from build123d import *
from OCP.BRepFilletAPI import BRepFilletAPI_MakeFillet

# Parameters (mm, degrees)
BOSS_EXTRUDE1_DEPTH = 5
BOSS_EXTRUDE2_DEPTH = 6.75
CHAMFER1_SIZE       = 3
CUT_EXTRUDE1_DEPTH  = 51.906134019
FILLET1_R1          = 1
FILLET1_R2          = 4
FILLET2_R           = 4
FILLET3_R           = 2
SKETCH5_R           = 1.25
CUT_EXTRUDE2_DEPTH  = 51.906134019
SKETCH6_R           = 1.25
CUT_EXTRUDE3_DEPTH  = 29.824774908
FILLET4_R           = 2
SKETCH7_R           = 3.5
CUT_EXTRUDE4_DEPTH  = 29.824774908
CHAMFER2_SIZE       = 0.5


with BuildPart() as part:
    # Sketch1 → Boss-Extrude1 (new, symmetric)
    with BuildSketch(Plane.XY):
        Polygon((-15, 33.787773645), (11.504683177, 39.681261814), (11.070572477, 41.63358041), (6.189775987, 40.548303662), (6.298303662, 40.060224013), (5.810224013, 39.951696338), (5.701696338, 40.439775987), (-11.855909094, 36.53572857), (-11.747381419, 36.047648921), (-12.235461068, 35.939121246), (-12.343988743, 36.427200895), (-17, 35.391906601), (-17, 20.3), (-16.5, 20.3), (-16.5, 19.8), (-17, 19.8), (-17, 17.5), (-15, 17.5), align=None)
    extrude(amount=BOSS_EXTRUDE1_DEPTH, both=True)

    # Sketch3 → Boss-Extrude2 (add, symmetric)
    with BuildSketch(Plane.XY):
        Polygon((-6.541001904, 35.668686722), (-6.975112604, 37.621005318), (-11.855909094, 36.53572857), (-11.747381419, 36.047648921), (-12.235461068, 35.939121246), (-12.343988743, 36.427200895), (-17, 35.391906601), (-17, 20.3), (-16.5, 20.3), (-16.5, 19.8), (-17, 19.8), (-17, 17.5), (-15, 17.5), (-15, 33.787773645), align=None)
    extrude(amount=BOSS_EXTRUDE2_DEPTH, both=True)

    # Chamfer1
    # the kernel refuses this chamfer: 3 mm, written as the material it takes off along each edge
    with BuildSketch(Plane(origin=(-4.866409254, 28.137569941, -6.75), x_dir=(0.0268403556117362, 0.005968127111591266, 0.9996219169112968), z_dir=(-0.21705534964808215, 0.9761592980600804, 0))) as chamfer1_piece_1_section:
        Polygon((CHAMFER1_SIZE * 0.999621916911, -CHAMFER1_SIZE * 0.0274958766106), (-CHAMFER1_SIZE * 0.0274958766106, -CHAMFER1_SIZE * 0.999621916911), (0, 0), align=None)
    chamfer1_piece_1 = extrude(amount=17.430097928, mode=Mode.PRIVATE)
    chamfer1_piece_1 = split(chamfer1_piece_1, bisect_by=Plane(origin=(-7.864790055, 36.398756806, -5), z_dir=(0, 0, -1)), keep=Keep.TOP, mode=Mode.PRIVATE)
    add(chamfer1_piece_1, mode=Mode.SUBTRACT)
    with BuildSketch(Plane(origin=(-4.866409254, 28.137569941, 6.75), x_dir=(-0.9757902287376033, -0.2169732846910676, 0.02749587661058649), z_dir=(-0.21705534964808215, 0.9761592980600804, 0))) as chamfer1_piece_2_section:
        Polygon((CHAMFER1_SIZE * 0.999621916911, -CHAMFER1_SIZE * 0.0274958766106), (-CHAMFER1_SIZE * 0.0274958766106, -CHAMFER1_SIZE * 0.999621916911), (0, 0), align=None)
    chamfer1_piece_2 = extrude(amount=17.430097928, mode=Mode.PRIVATE)
    chamfer1_piece_2 = split(chamfer1_piece_2, bisect_by=Plane(origin=(-7.864790055, 36.398756806, 5), z_dir=(0, 0, 1)), keep=Keep.TOP, mode=Mode.PRIVATE)
    add(chamfer1_piece_2, mode=Mode.SUBTRACT)

    # Sketch4 → Cut-Extrude1 (cut, through all)
    with BuildSketch(Plane.ZY.offset(17)):
        Polygon((-6.75, 30), (-3.75, 27), (-3.75, 17.5), (3.75, 17.5), (3.75, 27), (6.75, 30), (6.75, 0), (-6.75, 0), align=None)
    extrude(amount=-CUT_EXTRUDE1_DEPTH, mode=Mode.SUBTRACT)

    # Fillet1: one fillet with a radius per group of edges: ONE call of the kernel's fillet builder (fillet() takes one radius for all edges)
    fillet1_edges_1 = [part.edges().sort_by_distance(p)[0] for p in [
        (-9.686535148, 35.993679971, -6.75),
        (-9.686535148, 35.993679971, 6.75),
        (-16, 30, 6.75),
        (-16, 30, -6.75),
    ]]
    fillet1_edges_2 = [part.edges().sort_by_distance(p)[0] for p in [
        (-7.978256377, 36.373526833, 5),
        (-7.978256377, 36.373526833, -5),
        (-16, 27, -3.75),
        (-16, 27, 3.75),
    ]]
    fillet1 = BRepFilletAPI_MakeFillet(part.part.solid().wrapped)
    for e in fillet1_edges_1:
        fillet1.Add(FILLET1_R1, e.wrapped)
    for e in fillet1_edges_2:
        fillet1.Add(FILLET1_R2, e.wrapped)
    add(Compound.cast(fillet1.Shape()), mode=Mode.REPLACE)

    # Fillet2
    fillet2_edges = [part.edges().sort_by_distance(p)[0] for p in [
        (-15, 33.787773645, 0),
    ]]
    fillet(fillet2_edges, radius=FILLET2_R)

    # Fillet3
    fillet3_edges = [part.edges().sort_by_distance(p)[0] for p in [
        (-16, 17.5, -3.75),
        (-16, 17.5, 3.75),
    ]]
    fillet(fillet3_edges, radius=FILLET3_R)

    # Sketch5 → Cut-Extrude2 (cut, through all)
    with BuildSketch(Plane.ZY.offset(17)):
        with Locations(Location((0, 22.5, 0), (0, 0, 270))):
            Circle(SKETCH5_R)
    extrude(amount=-CUT_EXTRUDE2_DEPTH, mode=Mode.SUBTRACT)

    # Sketch6 → Cut-Extrude3 (cut, through all)
    with BuildSketch(Plane(origin=(-8.299779748, 37.326456989, 0), x_dir=(0.9761592980600814, 0.21705534964807782, 0), z_dir=(-0.21705534964807782, 0.9761592980600814, 0))):
        with Locations(Location((17.343433612, 0, 0), (0, 0, 180))):
            Circle(SKETCH6_R)
    extrude(amount=-CUT_EXTRUDE3_DEPTH, mode=Mode.SUBTRACT)

    # Fillet4
    fillet4_edges = [part.edges().sort_by_distance(p)[0] for p in [
        (11.287627827, 40.657421112, -5),
        (11.287627827, 40.657421112, 5),
    ]]
    fillet(fillet4_edges, radius=FILLET4_R)

    # Sketch7 → Cut-Extrude4 (cut, through all)
    with BuildSketch(Plane(origin=(-8.299779748, 37.326456989, 0), x_dir=(0.9761592980600813, 0.21705534964807838, 0), z_dir=(-0.21705534964807838, 0.9761592980600813, 0))):
        with Locations(Location((8.502484958, 0, 0), (0, 0, 180))):
            Circle(SKETCH7_R)
    extrude(amount=-CUT_EXTRUDE4_DEPTH, mode=Mode.SUBTRACT)

    # Chamfer2
    chamfer2_edges = [part.edges().sort_by_distance(p)[0] for p in [
        (3.850668243, 37.979341962, 0),
        (3.416557543, 39.931660559, 0),
    ]]
    chamfer(chamfer2_edges, length=CHAMFER2_SIZE)


solid = part.part
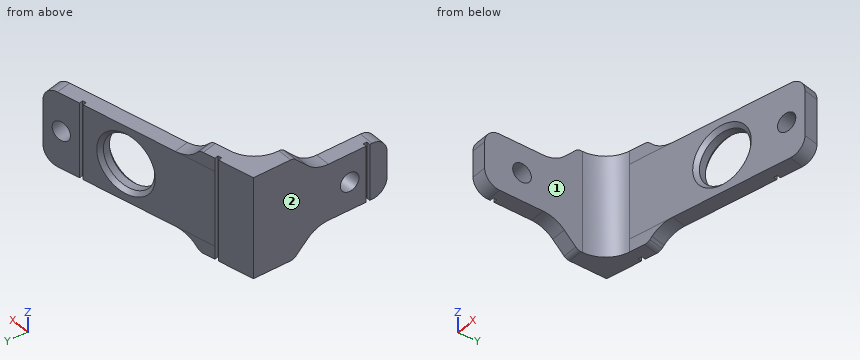
Source: CAD feature listing. Evaluate the final solid. Frame: model axes, mm. Face numbers are marked on the shaded views. A direction names the side the tool comes from. Round coordinates to 2 decimals unless told otherwise and drop trailing zeros. Loops run counter-clockwise (first coordinate to the right, second up) from the corner with the lowest first, then second, coordinate; pieces in that order, holes last. Notation, with made-up numbers: M 80.5,-19.75 L 100.5,-19.75 A15 cw 100.5,-11.75 Z; hole C 22,-13 d7. An arc over 180 degrees is marked long. Return JSON: item names as keys, results as strings. Group by question number.
1. Section query C-C on y = 29.25. Output: boundary loops of the cut face in (x, z).
2. Section query A-A on y = 22.5. Output: boundary loops of the cut face in (x, z), and give its area (3 significant figures).
3. Material intervals for line 1 along Z through (x, y) = (-16.2, 22.5); line 2 along X through (y, z) = (18.75, 2.25); line 3 along Y through (x, z) = (9.25, -2.25), sorted ascending. Write a range as from..to.
4. Pin query (flat end, axial travel): pin 1 (2 mm diameter, centred on x = -5, z = -1.5, fed in from +Y); pin 2 (1.6 mm diameter, centred on x = 4, y = 37.5, fed in from +Z); pin 3 (8 mm diameter, centred on x = -9, z = 5, fed in from +Y). Return the tip coordinate at first contact, or that it passes through.
5. Section query B-B on x = -10.75. Output: boundary loops of the cut face in (y, z), and give its area (3 significant figures).
6. Reachability of the marked faces 1 and 2 from +Z, -Z, +X, -X, +Y, -Y: full face, straight path, thin tool, end or side. Return the list, or none.
7. Section query D-D on z = 0. State how many separate pieces and enclosed holes the cut face has, and give its area (3 significant figures).
Checks:
{
 "1": {"outline": "M -17,-6 L -15,-6 L -15,6 L -17,6 Z"},
 "2": {"outline": "M -17,-3.75 L -15,-3.75 L -15,-1.25 L -17,-1.25 Z; M -17,1.25 L -15,1.25 L -15,3.75 L -17,3.75 Z", "area": "10.0 mm²"},
 "3": {"line 1": "z = -3.75..-1.25, 1.25..3.75", "line 2": "x = -17..-15", "line 3": "y = 39.18..41.23"},
 "4": {"pin 1": "stops at y = 38.28", "pin 2": "stops at z = 5", "pin 3": "stops at y = 38.06"},
 "5": {"outline": "M 34.73,-6.75 L 36.78,-6.75 L 36.78,6.75 L 34.73,6.75 Z", "area": "27.7 mm²"},
 "6": {"face 1": "+Z, -Z, +X, -Y", "face 2": "+Z, -Z, -X, +Y, -Y"},
 "7": {"separate pieces": "4", "enclosed holes": "0", "area": "66.9 mm²"}
}
